from build123d import *

# Parameters (mm, degrees)
F0_R     = 6.5
F1_DEPTH = 3
F2_R     = 2
F3_DEPTH = 4
F4_R     = 2.5
F5_DEPTH = 3
F6_R     = 6
F7_DEPTH = 2
F8_R     = 0.85
F9_DEPTH = 10.001


with BuildPart() as f1:
    # F0 (on Top) → F1 (new body)
    with BuildSketch(Plane.XY):
        Circle(F0_R)
    extrude(amount=F1_DEPTH)

    # F2 (on face) → F3 (join)
    with BuildSketch(Plane.XY.offset(3)):
        Circle(F2_R)
    extrude(amount=F3_DEPTH)

    # F4 (on face) → F5 (join)
    with BuildSketch(Plane.XY.offset(7)):
        Circle(F4_R)
    extrude(amount=F5_DEPTH)

    # F6 (on face) → F7 (cut)
    with BuildSketch(Plane(origin=(0, 0, 0), x_dir=(1, 0, 0), z_dir=(0, 0, -1))):
        Circle(F6_R)
    extrude(amount=-F7_DEPTH, mode=Mode.SUBTRACT)

    # F8 (on face) → F9 (cut, through all)
    with BuildSketch(Plane.XY.offset(10)):
        Circle(F8_R)
    extrude(amount=-F9_DEPTH, mode=Mode.SUBTRACT)


solid = f1.part
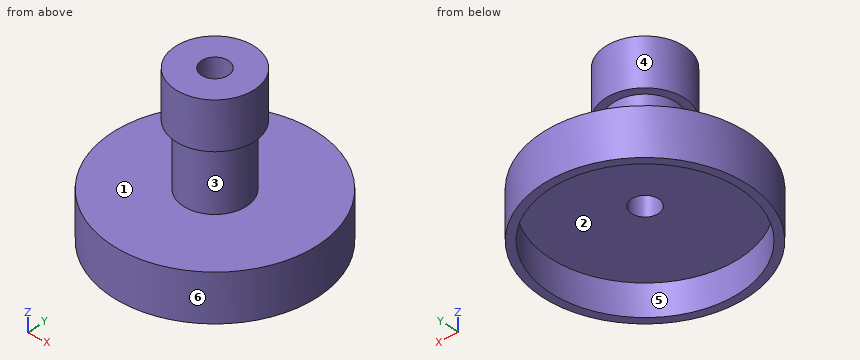
Here's how the part is built. I have some questions about the finished solid (model axes, mm). Face numbers are marked on the shaded views. A direction names the side the tool comes from. Give positions to 0.01 mm unless a question says otherwise; leave off trailing zeros. Order: outer loops, then holes, each group sorted by start corner. A loop starts at its lowest first (then second) coordinate and runs counter-clockwise, first axis right, second up. Notation, with made-up numbers: (48.25, 30) -> (90.25, 30) arc R13 cw to (90.25, 37) -> close; hole circle Ø8 at (38.25, 47). An arc over 180 degrees is marked (long way). Use a Markdown table: item, result. Add a question column.
Item 1: Imagine slicing it at C-C on z = 4.75. Please give me the cut outline in (x, y), plus the area to 3 significant figures.
Item 2: Imagine slicing it at A-A on x = 0. Please give me the cut outline in (y, z).
Item 3: Imagine slicing it at D-D on y = 5.75. Please give me the cut outline in (x, z), plus the area to 3 significant figures.
Item 4: Will these pins go through, and if not, where does the flat tip stop? pin 1 (6 mm diameter, centred on x = 4.5, y = -4.5, fed in from +Z); pin 2 (2.5 mm diameter, centred on x = -0.5, y = 0.5, fed in from -Z); pin 3 (1.5 mm diameter, centred on x = 0.5, z = 9, fed in from +Y).
Item 5: For the marked faces 4, 5 and 6, which set-ups out of +Z, -Z, +X, -X, +Y, -Y let a thin tool reach every point of the face, with its end or its side?
Item 6: If we mould it in two halves opening along Y, with no side actions, what happens to the marked faces 1, 2 and 3? For each: pulls with the +Y half, pulls with the -Y half, needs draft (parallel to the pull), parting line crosses it, or undercut.
Item 7: I need wall thicknesses on line 1 (Y direction, x = 0, z = 8); line 2 (Z direction, x = 1.75, y = -1.5); line 3 (Y direction, x = 0, z = 4.25). Which ranges of each line are inside material? Lowest first, please.
Data:
| question | item | result |
|---|---|---|
| 1 | outline | circle Ø4 at (0, 0); hole circle Ø1.7 at (0, 0) |
| 1 | area | 10.3 mm² |
| 2 | outline | (-6.5, 0) -> (-6, 0) -> (-6, 2) -> (-0.85, 2) -> (-0.85, 10) -> (-2.5, 10) -> (-2.5, 7) -> (-2, 7) -> (-2, 3) -> (-6.5, 3) -> close; (0.85, 2) -> (6, 2) -> (6, 0) -> (6.5, 0) -> (6.5, 3) -> (2, 3) -> (2, 7) -> (2.5, 7) -> (2.5, 10) -> (0.85, 10) -> close |
| 3 | outline | (-3.03, 0) -> (-1.71, 0) -> (-1.71, 2) -> (1.71, 2) -> (1.71, 0) -> (3.03, 0) -> (3.03, 3) -> (-3.03, 3) -> close |
| 3 | area | 11.3 mm² |
| 4 | pin 1 | stops at z = 3 |
| 4 | pin 2 | stops at z = 2 |
| 4 | pin 3 | stops at y = 2.5 |
| 5 | face 4 | +Z |
| 5 | face 5 | -Z |
| 5 | face 6 | +Z, -Z |
| 6 | face 1 | needs draft |
| 6 | face 2 | undercut |
| 6 | face 3 | parting line crosses it |
| 7 | line 1 | y = -2.5 to -0.85, 0.85 to 2.5 |
| 7 | line 2 | z = 2 to 3, 7 to 10 |
| 7 | line 3 | y = -2 to -0.85, 0.85 to 2 |
